For this review, take the finished solid that the model builds, in its own axes (mm). A direction names the side the tool comes from. Coordinates: 2 decimals unless noted, no trailing zeros. Loops run counter-clockwise (first coordinate to the right, second up) from the corner with the lowest first, then second, coordinate; pieces in that order, holes last. Notation, with made-up numbers: M -38,1.25 L -15,1.25 A17 cw -15,25.25 Z; hole C 35.25,5.5 d3. An arc over 180 degrees is marked long. Use one line per item in the form item = value.
```python
from build123d import *

# Parameters (mm, degrees)
SKETCH1_R               = 14.2875
BOSS_EXTRUDE1_DEPTH     = 40
CUT_EXTRUDE1_REACH      = 46.814
SKETCH2_R               = 6.3754
SKETCH3_R               = 7.9629
CUT_EXTRUDE2_DEPTH      = 20
CUT_EXTRUDE3_DEPTH      = 20
CUT_EXTRUDE4_REACH      = 46.814
CUT_EXTRUDE4_END_RADIUS = 14.2875
SKETCH5_R               = 2
CIRPATTERN1_COUNT       = 2
CIRPATTERN1_ANGLE       = 90


with BuildPart() as part:
    # Sketch1 → Boss-Extrude1 (new body)
    with BuildSketch(Plane(origin=(0, 0, 0), x_dir=(1, 0, 0), z_dir=(0, 1, 0))):
        with Locations(Location((0, 0, 0), (0, 0, 270))):
            Circle(SKETCH1_R)
    extrude(amount=BOSS_EXTRUDE1_DEPTH)

    # Sketch2 → Cut-Extrude1 (cut, up to next)
    with BuildSketch(Plane(origin=(0, 0, 0), x_dir=(-1, 0, 0), z_dir=(0, -1, 0)), mode=Mode.PRIVATE) as cut_extrude1_sk1:
        with Locations(Location((0, 0, 0), (0, 0, 90))):
            Circle(SKETCH2_R)
    cut_extrude1_tool1 = extrude(cut_extrude1_sk1.sketch, amount=-CUT_EXTRUDE1_REACH, mode=Mode.PRIVATE) & part.part
    add(cut_extrude1_tool1.solids().sort_by_distance((0, 0, 0))[0], mode=Mode.SUBTRACT)

    # Sketch3 → Cut-Extrude2 (cut)
    with BuildSketch(Plane(origin=(0, 40, 0), x_dir=(1, 0, 0), z_dir=(0, 1, 0))):
        with Locations(Location((0, 0, 0), (0, 0, 270))):
            Circle(SKETCH3_R)
    extrude(amount=-CUT_EXTRUDE2_DEPTH, mode=Mode.SUBTRACT)

    # Sketch4 → Cut-Extrude3 (cut)
    with BuildSketch(Plane(origin=(0, 40, 0), x_dir=(1, 0, 0), z_dir=(0, 1, 0))):
        with BuildLine():
            Line((2.625, -10), (-2.625, -10))
            Line((-2.625, -10), (-2.625, -7.517788997))
            ThreePointArc((-2.625, -7.517788997), (0, -7.9629), (2.625, -7.517788997))
            Line((2.625, -7.517788997), (2.625, -10))
        make_face()
    extrude(amount=-CUT_EXTRUDE3_DEPTH, mode=Mode.SUBTRACT)

    # Cut-Extrude4: up to this cylinder (the profile starts inside it)
    cut_extrude4_end = Plane(origin=(0, 20, 0), z_dir=(0, -1, 0)) * Cylinder(CUT_EXTRUDE4_END_RADIUS, 150.503, mode=Mode.PRIVATE)
    # Sketch5 → Cut-Extrude4 (cut, up to the surface)
    with BuildSketch(Plane.XY, mode=Mode.PRIVATE) as cut_extrude4_sk1:
        with Locations(Location((0, 33.65, 0), (0, 0, 180))):
            Circle(SKETCH5_R)
    cut_extrude4_tool1 = extrude(cut_extrude4_sk1.sketch, amount=CUT_EXTRUDE4_REACH, mode=Mode.PRIVATE) & cut_extrude4_end
    # Sketch5 → Cut-Extrude4 (cut, up to the surface)
    with BuildSketch(Plane.XY, mode=Mode.PRIVATE) as cut_extrude4_sk2:
        with Locations(Location((0, 6.35, 0), (0, 0, 180))):
            Circle(SKETCH5_R)
    cut_extrude4_tool2 = extrude(cut_extrude4_sk2.sketch, amount=CUT_EXTRUDE4_REACH, mode=Mode.PRIVATE) & cut_extrude4_end
    cut_extrude4 = cut_extrude4_tool1.solids().sort_by_distance((0, 33.65, 0))[0] + cut_extrude4_tool2.solids().sort_by_distance((0, 6.35, 0))[0]
    add(cut_extrude4, mode=Mode.SUBTRACT)

    # CirPattern1: Cut-Extrude4 ×2 about axis
    cirpattern1_axis = Axis((0, 40, 0), (0, 1, 0))
    for i in range(1, CIRPATTERN1_COUNT):
        add(cut_extrude4.rotate(cirpattern1_axis, i * CIRPATTERN1_ANGLE / (CIRPATTERN1_COUNT - 1)), mode=Mode.SUBTRACT)


solid = part.part
```
1. Consider section D-D on z = 3. Write out the cut boundary in (x, y).
Computed values:
outline = M -13.97,0 L -5.63,0 L -5.63,20 L -7.38,20 L -7.38,40 L -13.97,40 Z; M 5.63,0 L 13.97,0 L 13.97,40 L 7.38,40 L 7.38,20 L 5.63,20 Z
2. Draft analysis for pull direction X (two halves, no side actions). For faces 5 (the face through (-13.948, 19.72, -3.097)), 6 (the face through (0, 30, 10)), 7 (the face through (-0.923, 35.424, 12.114)), 8 (the face through (10.109, 4.367, -0.26)), state which applies: +X half, -X half, draft (parallel to the pull), parting line (faces both ways), or undercut.
Computed values:
face_5 = parting line
face_6 = undercut
face_7 = undercut
face_8 = draft
3. Tool access review of faces 1 (the face through (10.948, 35.424, 0.923)), 2 (the face through (0.26, 4.367, 10.113)), 3 (the face through (-1.73, 20, 6.3)), 4 (the face through (-6, 40, 6)): name each direction out of +Z, -Z, +X, -X, +Y, -Y from which nothing blocks a thin tool from reaching the whole face with its end or side.
Computed values:
face_1 = +X
face_2 = +Z
face_3 = +Y
face_4 = +Z, -Z, +X, -X, +Y
4. Consider section A-A on x = 0. Write out the cut boundary in (y, z).
Computed values:
outline = M 0,-14.29 L 40,-14.29 L 40,-7.96 L 20,-7.96 L 20,-6.38 L 0,-6.38 Z; M 0,6.38 L 4.35,6.38 L 4.35,14.29 L 0,14.29 Z; M 8.35,6.38 L 20,6.38 L 20,10 L 31.65,10 L 31.65,14.29 L 8.35,14.29 Z; M 35.65,10 L 40,10 L 40,14.29 L 35.65,14.29 Z
5. For pin 1 Ø10 at (x, y) = (6.5, 22.5) entering from -Z; pin 2 Ø5 at (y, z) = (33.65, 0) entering from +X; pin 3 Ø5 at (x, y) = (4.5, 17.5) entering from -Z; pin 4 Ø8 at (y, z) = (21, 5.5) entering from +X, all flat-tipped, find the tip position at first contact; note any pin that passes through.
Computed values:
pin_1 = -14.21
pin_2 = 14.29
pin_3 = -14.15
pin_4 = 14.21
6. Consider section B-B on z = 0. Write out the cut boundary in (x, y).
Computed values:
outline = M -14.29,0 L -6.38,0 L -6.38,20 L -7.96,20 L -7.96,40 L -14.29,40 Z; M 6.38,0 L 14.29,0 L 14.29,4.35 L 6.38,4.35 Z; M 6.38,8.35 L 14.29,8.35 L 14.29,31.65 L 7.96,31.65 L 7.96,20 L 6.38,20 Z; M 7.96,35.65 L 14.29,35.65 L 14.29,40 L 7.96,40 Z
7. Wall thickness on line 1 along Y through (x, z) = (0, 11.25); line 2 along X through (y, z) = (15, 0); line 3 along X through (y, z) = (28.75, 0): over which ranges is each line inside the solid? List them lowest first. Write a range as from..to.
Computed values:
line_1 = 0..4.35, 8.35..31.65, 35.65..40
line_2 = -14.29..-6.38, 6.38..14.29
line_3 = -14.29..-7.96, 7.96..14.29
8. Consider section C-C on y = 33. Write out the cut boundary in (x, z) (1 decimal), plus the area to 3 significant figures.
Computed values:
outline = M -2.6,7.5 L -2.6,10 L -1.9,10 L -1.9,14.2 A14.3 ccw long 14.2,-1.9 L 7.7,-1.9 A8 cw long Z; M 1.9,10 L 2.6,10 L 2.6,7.5 A8 cw 7.7,1.9 L 14.2,1.9 A14.3 ccw 1.9,14.2 Z
area = 391 mm2
